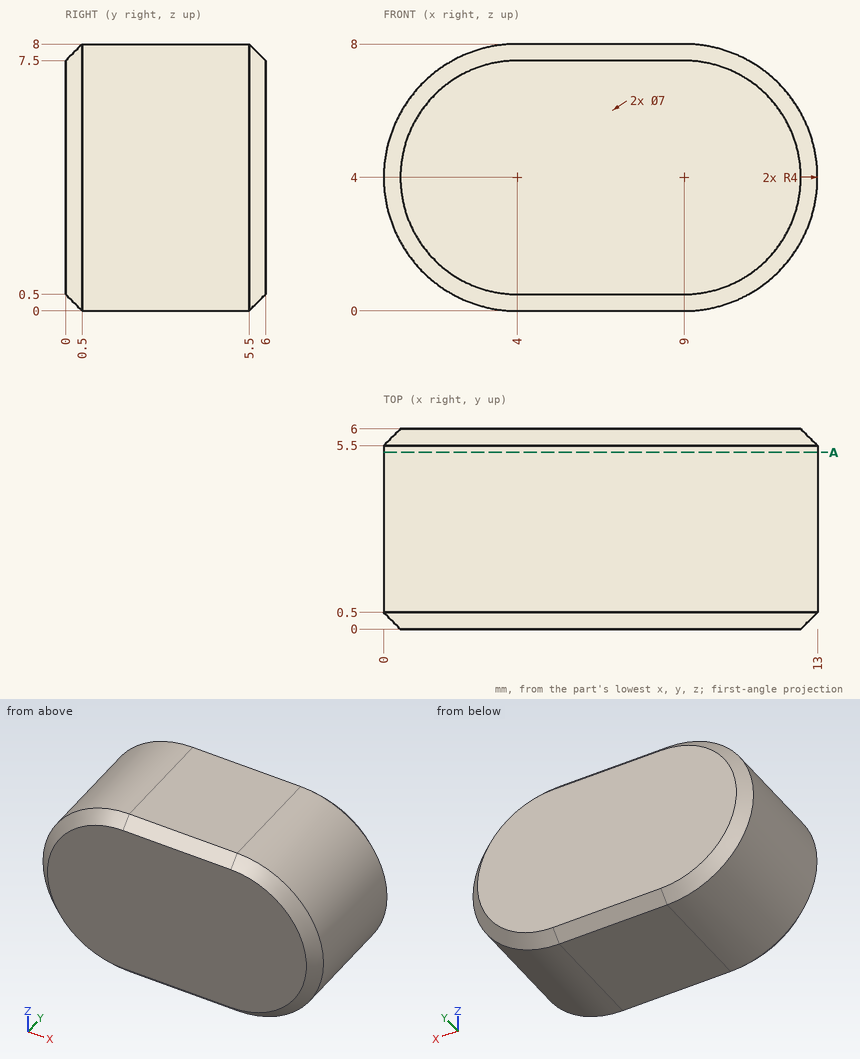
Study the drawing (mm; zero at the part's minimum x, y, z) and answer. Round coordinates to 2 decimals unless told otherwise and drop trailing zeros. Write each loop counter-clockwise with the first axis right and the second up, starting at its lowest first coordinate (ties: lowest second). Pieces come first, ordered by that corner, then holes.
1) Given pin 1 Ø1 at (y, z) = (3.5, 1) entering from -X; pin 2 Ø3 at (x, y) = (11, 4) entering from +Z, each flat-ended and moving along its own axis, determine where each tip first touches the part or whether it passes through.
2) A cutting plane is placed at A-A (y = 5.3). Give the vertices of the cut face in (x, z).
3) Straight lines are drawn through the part: line 1 (X direction, y = 0.35, z = 2); line 2 (X direction, y = 1.95, z = 7.5); line 3 (Z direction, x = 8.5, y = 5.65). For each, find the intervals that lie inside material, in ascending order.
Completed:
1. pin 1: stops at x = 0.88
1. pin 2: stops at z = 7.97
2. outline: (4, 0) - (9, 0) arc R4 ccw to (9, 8) - (4, 8) arc R4 ccw to start
3. line 1: x = 0.71 to 12.29
3. line 2: x = 2.06 to 10.94
3. line 3: z = 0.15 to 7.85
